from build123d import *

# Parameters (mm, degrees)
Y_KSEKLIK_EKSTR_ZYON1_DEPTH = 250
IZIM3_R                     = 7.5
Y_KSEKLIK_EKSTR_ZYON3_DEPTH = 15


with BuildPart() as part:
    # Çizim2 → Yükseklik-Ekstrüzyon1 (new body, symmetric)
    with BuildSketch(Plane.XY):
        Polygon((10, 25), (40, 25), (40, 0), (-40, 0), (-40, 25), (-10, 25), (-10, 20), (10, 20), align=None)
    extrude(amount=Y_KSEKLIK_EKSTR_ZYON1_DEPTH, both=True)

    # Çizim3 → Yükseklik-Ekstrüzyon3 (add)
    with BuildSketch(Plane(origin=(40, 0, 0), x_dir=(0, 0, -1), z_dir=(1, 0, 0))):
        with BuildLine():
            Line((-20, 25), (20, 25))
            Line((20, 25), (20, 87.5))
            ThreePointArc((20, 87.5), (0, 107.5), (-20, 87.5))
            Line((-20, 87.5), (-20, 25))
        make_face()
        with Locations((0, 87.5)):
            Circle(IZIM3_R, mode=Mode.SUBTRACT)
    y_kseklik_ekstr_zyon3 = extrude(amount=-Y_KSEKLIK_EKSTR_ZYON3_DEPTH)

    # Aynalama1: Yükseklik-Ekstrüzyon3 across plane
    add(y_kseklik_ekstr_zyon3.mirror(Plane.ZY))


solid = part.part
Verification items for the finished model (mm, model axes). A direction names the side the tool comes from. Give positions to 0.01 mm unless a question says otherwise; leave off trailing zeros. Order: outer loops, then holes, each group sorted by start corner. A loop starts at its lowest first (then second) coordinate and runs counter-clockwise, first axis right, second up. Notation, with made-up numbers: M -2.75,-7 L 41.25,-7 A23 ccw 41.25,24 Z; hole C 13,50.5 d1. An arc over 180 degrees is marked long. Answer as a JSON object with one key per item and string values. Group by question number.
1) Access from +Z, -Z, +X, -X, +Y, -Y to the whole of each face (thin tool, end or side, straight path). Record for faces 1 (the face through (-32.605, 107.495, -0.44)), 2 (the face through (33, 56, -20)), 3 (the face through (-33, 57, 20)), 4 (the face through (-40, 26, 1)), 5 (the face through (-25, 67, 0)).
2) Cross-section at C-C (x = -20.5). Enter the section's corners in (y, z), then the cut area to 3 significant figures.
3) Scan lines: line 1 along X through (y, z) = (61, -4); line 2 along Y through (x, z) = (-31.5, 0); line 3 along Z through (x, y) = (28, 87). Record each from-to range of solid material in increasing order. Write a range as [from, to].
4) Depth check by flat-ended pin: pin 1 Ø4.5 at (x, y) = (29, 47.5) entering from +Z; pin 2 Ø1.5 at (x, z) = (-10.5, -89.5) entering from +Y; pin 3 Ø7.5 at (x, y) = (31.5, 44.5) entering from -Z. Enter the tip coordinate at first touch or a pass-through.
5) Cross-section at B-B (z = 83). Enter the section's corners in (x, y).
6) Mould release check, pull along Y, two halves, no side actions. Record for faces 6 (the face through (32.605, 107.495, -0.44)), 7 (the face through (32.61, 80.18, 1.63)), 8 (the face through (33, 57, 20)), 9 (the face through (-32.61, 80.18, 1.63)): released by +Y, released by -Y, zero draft, split by the parting line, or undercut.
7) Cross-section at A-A (z = 0). Enter the section's corners in (x, y).
Result sheet:
{
 "1": {"face 1": "+X, -X, +Y", "face 2": "-Z, +X, -X, +Y", "face 3": "+Z, +X, -X, +Y", "face 4": "+Z, -Z, -X, +Y, -Y", "face 5": "+Z, -Z, +Y"},
 "2": {"outline": "M 0,-250 L 25,-250 L 25,250 L 0,250 Z", "area": "12,500 mm2"},
 "3": {"line 1": "x = [-40, -25], [25, 40]", "line 2": "y = [0, 80], [95, 107.5]", "line 3": "z = [-20, -7.48], [7.48, 20]"},
 "4": {"pin 1": "stops at z = 20", "pin 2": "stops at y = 25", "pin 3": "stops at z = -20"},
 "5": {"outline": "M -40,0 L 40,0 L 40,25 L 10,25 L 10,20 L -10,20 L -10,25 L -40,25 Z"},
 "6": {"face 6": "released by +Y", "face 7": "undercut", "face 8": "zero draft", "face 9": "undercut"},
 "7": {"outline": "M -40,0 L 40,0 L 40,80 L 25,80 L 25,25 L 10,25 L 10,20 L -10,20 L -10,25 L -25,25 L -25,80 L -40,80 Z; M -40,95 L -25,95 L -25,107.5 L -40,107.5 Z; M 25,95 L 40,95 L 40,107.5 L 25,107.5 Z"}
}
